```python
from build123d import *

# Parameters (mm, degrees)
F0_R     = 25
F1_DEPTH = 40
F3_DEPTH = 25


with BuildPart() as f1:
    # F0 (on Front) → F1 (new body)
    with BuildSketch(Plane.XZ):
        Circle(F0_R)
    extrude(amount=-F1_DEPTH)

    # F2 (on Front) → F3 (cut)
    with BuildSketch(Plane.XZ):
        Polygon((5.559986, 9.630178), (-5.559986, 9.630178), (-11.119972, 0), (-5.559986, -9.630178), (5.559986, -9.630178), (11.119972, 0), align=None)
    extrude(amount=-F3_DEPTH, mode=Mode.SUBTRACT)


solid = f1.part
```
Design review of the part built by this model. Coordinates are the model's own, in mm. A direction names the side the tool comes from. Coordinates: 2 decimals unless noted, no trailing zeros. Order: outer loops, then holes, each group sorted by start corner. A loop starts at its lowest first (then second) coordinate and runs counter-clockwise, first axis right, second up. Notation, with made-up numbers: (77.25, 85.5) - (110.25, 85.5) arc R29 ccw to (110.25, 118.5) - close; hole circle Ø3 at (9.25, -33). An arc over 180 degrees is marked (long way). One line per question, with ' | ' between items.
Q1. For faces 1 (the flat face through (0, 0, -11)), 2 (the flat face through (8.379, 12.325, 4.748)), list the 3-axis set-ups (+Z, -Z, +X, -X, +Y, -Y) from which the entire face can be reached by the end or side of a thin tool; tool diameter is ignored.
Answer key:
face 1: +Z, -Z, +X, -X, -Y | face 2: -Y
Q2. Consider section A-A, the plane y = 15. Give the boundary of the cut face in (x, z), then the cut area to 3 significant figures.
Answer key:
outline: circle Ø50 at (0, 0); hole (-11.12, 0) - (-5.56, -9.63) - (5.56, -9.63) - (11.12, 0) - (5.56, 9.63) - (-5.56, 9.63) - close | area: 1,640 mm2
Q3. To check wall thickness, follow line 1 along X through (y, z) = (22, -1.5); line 2 along Z through (x, y) = (-4, 16); line 3 along Z through (x, y) = (4.5, 7). State the ranges of each line that lie inside material, in increasing order.
Answer key:
line 1: x = -24.95 to -10.25, 10.25 to 24.95 | line 2: z = -24.68 to -9.63, 9.63 to 24.68 | line 3: z = -24.59 to -9.63, 9.63 to 24.59
Q4. Consider section C-C, the plane y = 37. Give the boundary of the cut face in (x, z), then the cut area to 3 significant figures.
Answer key:
outline: circle Ø50 at (0, 0) | area: 1,960 mm2
Q5. Clearance check with flat-ended pins moving along their axes: pin 1 Ø3.5 at (x, y) = (1, 13.5) entering from +Z; pin 2 Ø6 at (x, z) = (0.5, -0.5) entering from -Y; pin 3 Ø3 at (x, y) = (-13, 33) entering from +Z. State where each tip first meets the part, or that it passes through.
Answer key:
pin 1: stops at z = 25 | pin 2: stops at y = 25 | pin 3: stops at z = 22.2
Q6. Consider section D-D, the plane z = 18. Give the boundary of the cut face in (x, y), then the cut area to 3 significant figures.
Answer key:
outline: (-17.35, 0) - (17.35, 0) - (17.35, 40) - (-17.35, 40) - close | area: 1,390 mm2
Q7. Consider section B-B, the plane x = 0. Give the boundary of the cut face in (y, z).
Answer key:
outline: (0, -25) - (40, -25) - (40, 25) - (0, 25) - (0, 9.63) - (25, 9.63) - (25, -9.63) - (0, -9.63) - close
